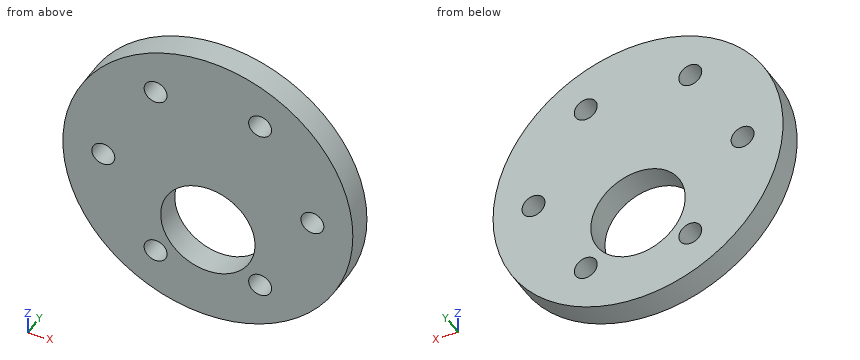
```python
from build123d import *

# Parameters (mm, degrees)
SKETCH3_R           = 21.5
SKETCH3_R_2         = 7
BOSS_EXTRUDE1_DEPTH = 4
SKETCH3_4_R         = 1.7
CUT_EXTRUDE2_DEPTH  = 4
CIRPATTERN1_COUNT   = 6


with BuildPart() as part:
    # Sketch3 → Boss-Extrude1 (new body)
    with BuildSketch(Plane(origin=(0, 0, 0), x_dir=(1, 0, 0), z_dir=(0, 1, 0))):
        Circle(SKETCH3_R)
        with Locations((0, 7)):
            Circle(SKETCH3_R_2, mode=Mode.SUBTRACT)
    extrude(amount=BOSS_EXTRUDE1_DEPTH)

    # Sketch3<4> → Cut-Extrude2 (cut)
    with BuildSketch(Plane(origin=(0, 0, 0), x_dir=(1, 0, 0), z_dir=(0, 1, 0))):
        with Locations((-15.5, 0)):
            Circle(SKETCH3_4_R)
    cut_extrude2 = extrude(amount=CUT_EXTRUDE2_DEPTH, mode=Mode.SUBTRACT)

    # CirPattern1: Cut-Extrude2 ×6 about axis
    cirpattern1_axis = Axis((0, 0, 0), (0, 1, 0))
    for i in range(1, CIRPATTERN1_COUNT):
        add(cut_extrude2.rotate(cirpattern1_axis, i * 360 / CIRPATTERN1_COUNT), mode=Mode.SUBTRACT)


solid = part.part
```
Check sheet for the modelled part. Datum: model origin and axes. Units: mm. Round coordinates to 2 decimals unless told otherwise and drop trailing zeros. Loops run counter-clockwise (first coordinate to the right, second up) from the corner with the lowest first, then second, coordinate; pieces in that order, holes last. Notation, with made-up numbers: (-24, 9) -> (-1, 9) arc R13 ccw to (-1, 24) -> close; hole circle Ø9 at (-21, -21.5). An arc over 180 degrees is marked (long way). Write item = value, one per line. Start each with the question number.
1) Gauge pin test, flat ends, axial feed: pin 1 Ø2.5 at (x, z) = (7.75, -13.42) entering from +Y; pin 2 Ø2 at (y, z) = (2.5, 4) entering from -X; pin 3 Ø2 at (x, y) = (-12, 2) entering from -Z; pin 4 Ø1.5 at (x, y) = (-3, 1) entering from +Z. Record the tip position at first contact, or that the pin passes through.
2) Sectioned sample at D-D, the plane y = 1.35. Record the cut outline in (x, z), plus the area to 3 significant figures.
3) Sectioned sample at A-A, the plane z = -7. Record the cut outline in (x, y), plus the area to 3 significant figures.
4) Sectioned sample at B-B, the plane x = 0. Record the cut outline in (y, z).
5) Sectioned sample at C-C, the plane z = 14. Record the cut outline in (x, y), plus the area to 3 significant figures.
6) Thickness scan on probe 1 along X at (y, z) = (1, 13.5); probe 2 along X at (y, z) = (2.7, -1.5); probe 3 along X at (y, z) = (0.5, -13). Record the ranges inside material, lowest first.
Results are:
q1.pin_1 = through
q1.pin_2 = -21.29
q1.pin_3 = -18.47
q1.pin_4 = 21.38
q2.outline = circle Ø43 at (0, 0); hole circle Ø3.4 at (-15.5, 0); hole circle Ø3.4 at (-7.75, -13.42); hole circle Ø3.4 at (-7.75, 13.42); hole circle Ø14 at (0, -7); hole circle Ø3.4 at (7.75, -13.42); hole circle Ø3.4 at (7.75, 13.42); hole circle Ø3.4 at (15.5, 0)
q2.area = 1,240 mm^2
q3.outline = (-20.33, 0) -> (-7, 0) -> (-7, 4) -> (-20.33, 4) -> close; (7, 0) -> (20.33, 0) -> (20.33, 4) -> (7, 4) -> close
q3.area = 107 mm^2
q4.outline = (0, -21.5) -> (4, -21.5) -> (4, -14) -> (0, -14) -> close; (0, 0) -> (4, 0) -> (4, 21.5) -> (0, 21.5) -> close
q5.outline = (-16.32, 0) -> (-9.35, 0) -> (-9.35, 4) -> (-16.32, 4) -> close; (-6.15, 0) -> (6.15, 0) -> (6.15, 4) -> (-6.15, 4) -> close; (9.35, 0) -> (16.32, 0) -> (16.32, 4) -> (9.35, 4) -> close
q5.area = 105 mm^2
q6.probe_1 = -16.73 to -9.45, -6.05 to 6.05, 9.45 to 16.73
q6.probe_2 = -21.45 to -16.3, -14.7 to -4.33, 4.33 to 14.7, 16.3 to 21.45
q6.probe_3 = -17.12 to -9.4, -6.1 to -3.61, 3.61 to 6.1, 9.4 to 17.12
